Verification items for this drawing (mm, ordinates from the low corner). A direction names the side the tool comes from. Give positions to 0.01 mm unless a question says otherwise; leave off trailing zeros. Order: outer loops, then holes, each group sorted by start corner. A loop starts at its lowest first (then second) coordinate and runs counter-clockwise, first axis right, second up.
(1) Mould release check, pull along Y, two halves, no side actions. Record for the marked faces 3, 4 and 5: pulls with the +Y half, pulls with the -Y half, needs draft (parallel to the pull), parting line crosses it, or undercut.
(2) Sectioned sample at C-C on z = 5.5. Record the cut outline in (x, y).
(3) Sectioned sample at B-B on y = 6. Record the cut outline in (x, z).
(4) Gauge pin test, flat end, axial feed: pin 1 (1.5 mm diameter, centred on x = 3.5, y = 6.5, fed in from +Z). Record the tip position at first contact, or that the pin passes through.
(5) Scan lines: L1, parallel to Y at x = 2, z = 5; L2, parallel to X at y = 2.5, z = 2.5; L3, parallel to Z at x = 10.25, y = 4.5. Record each from-to range of solid material in increasing order.
(6) Sectioned sample at A-A on x = 2. Record the cut outline in (y, z).
(7) Sectioned sample at D-D on y = 1.25. Record the cut outline in (x, z), plus the area to 3 significant figures.
(8) Access from +Z, -Z, +X, -X, +Y, -Y to the whole of each face (thin tool, end or side, straight path). Record for the marked faces 1 and 2.
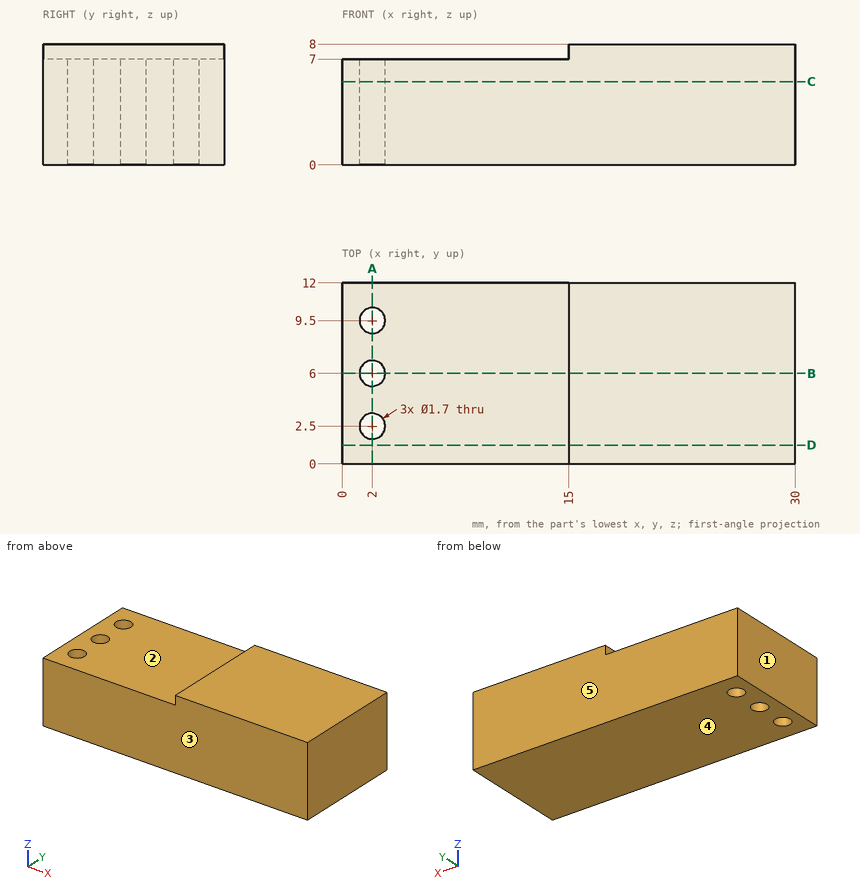
Ans:
1. face 3: pulls with the -Y half
1. face 4: needs draft
1. face 5: pulls with the +Y half
2. outline: (0, 0) - (30, 0) - (30, 12) - (0, 12) - close; hole circle Ø1.7 at (2, 2.5); hole circle Ø1.7 at (2, 6); hole circle Ø1.7 at (2, 9.5)
3. outline: (0, 0) - (1.15, 0) - (1.15, 7) - (0, 7) - close; (2.85, 0) - (30, 0) - (30, 8) - (15, 8) - (15, 7) - (2.85, 7) - close
4. pin 1: stops at z = 7
5. L1: y = 0 to 1.65, 3.35 to 5.15, 6.85 to 8.65, 10.35 to 12
5. L2: x = 0 to 1.15, 2.85 to 30
5. L3: z = 0 to 7
6. outline: (0, 0) - (1.65, 0) - (1.65, 7) - (0, 7) - close; (3.35, 0) - (5.15, 0) - (5.15, 7) - (3.35, 7) - close; (6.85, 0) - (8.65, 0) - (8.65, 7) - (6.85, 7) - close; (10.35, 0) - (12, 0) - (12, 7) - (10.35, 7) - close
7. outline: (0, 0) - (30, 0) - (30, 8) - (15, 8) - (15, 7) - (0, 7) - close
7. area: 225 mm2
8. face 1: +Z, -Z, -X, +Y, -Y
8. face 2: +Z, -X, +Y, -Y
